from build123d import *

# Parameters (mm, degrees)
CROQUIS1_W              = 48
CROQUIS1_H              = 46
SALIENTE_EXTRUIR1_DEPTH = 26
CROQUIS2_W              = 44
CROQUIS2_H              = 22
CORTAR_EXTRUIR1_DEPTH   = 46
CROQUIS3_W              = 12.57
CROQUIS3_H              = 22
CORTAR_EXTRUIR3_DEPTH   = 60.236812878
REDONDEO3_R             = 10
REDONDEO4_R             = 10
CROQUIS16_W             = 12.57
CROQUIS16_H             = 4
CORTAR_EXTRUIR19_DEPTH  = 10.25
CROQUIS21_W             = 12.57
CROQUIS21_H             = 4
CORTAR_EXTRUIR20_DEPTH  = 10.25
CORTAR_EXTRUIR21_DEPTH  = 10.25
CROQUIS23_R             = 2.5
CORTAR_EXTRUIR22_DEPTH  = 53


with BuildPart() as part:
    # Croquis1 → Saliente-Extruir1 (new body)
    with BuildSketch(Plane(origin=(0, 0, 0), x_dir=(1, 0, 0), z_dir=(0, 1, 0))):
        Rectangle(CROQUIS1_W, CROQUIS1_H)
    extrude(amount=-SALIENTE_EXTRUIR1_DEPTH)

    # Croquis2 → Cortar-Extruir1 (cut)
    with BuildSketch(Plane.XY.offset(23)):
        with Locations((0, -15)):
            Rectangle(CROQUIS2_W, CROQUIS2_H)
    extrude(amount=-CORTAR_EXTRUIR1_DEPTH, mode=Mode.SUBTRACT)

    # Croquis3 → Cortar-Extruir3 (cut, through all)
    with BuildSketch(Plane(origin=(24, 0, 0), x_dir=(0, 0, -1), z_dir=(1, 0, 0))):
        with Locations((-16.715, -15)):
            Rectangle(CROQUIS3_W, CROQUIS3_H)
        with Locations((16.715, -15)):
            Rectangle(CROQUIS3_W, CROQUIS3_H)
    extrude(amount=-CORTAR_EXTRUIR3_DEPTH, mode=Mode.SUBTRACT)

    # Redondeo3
    redondeo3_edges = [part.edges().sort_by_distance(p)[0] for p in [
        (23, -26, 10.43),
        (23, -26, -10.43),
    ]]
    fillet(redondeo3_edges, radius=REDONDEO3_R)

    # Redondeo4
    redondeo4_edges = [part.edges().sort_by_distance(p)[0] for p in [
        (-23, -26, 10.43),
        (-23, -26, -10.43),
    ]]
    fillet(redondeo4_edges, radius=REDONDEO4_R)

    # Croquis16 → Cortar-Extruir19 (cut)
    with BuildSketch(Plane.ZY.offset(24)):
        with Locations((-16.715, -2)):
            Rectangle(CROQUIS16_W, CROQUIS16_H)
        with Locations((16.715, -2)):
            Rectangle(CROQUIS16_W, CROQUIS16_H)
    extrude(amount=-CORTAR_EXTRUIR19_DEPTH, mode=Mode.SUBTRACT)

    # Croquis21 → Cortar-Extruir20 (cut)
    with BuildSketch(Plane(origin=(24, 0, 0), x_dir=(0, 0, -1), z_dir=(1, 0, 0))):
        with Locations((-16.715, -2)):
            Rectangle(CROQUIS21_W, CROQUIS21_H)
        with Locations((16.715, -2)):
            Rectangle(CROQUIS21_W, CROQUIS21_H)
    extrude(amount=-CORTAR_EXTRUIR20_DEPTH, mode=Mode.SUBTRACT)

    # Croquis22 → Cortar-Extruir21 (cut)
    with BuildSketch(Plane(origin=(0, 0, 0), x_dir=(1, 0, 0), z_dir=(0, 1, 0))):
        with BuildLine():
            Line((13.75, -10.43), (13.75, -23))
            Line((13.75, -23), (-13.75, -23))
            Line((-13.75, -23), (-13.75, -10.43))
            ThreePointArc((-13.75, -10.43), (0, -17.258255995), (13.75, -10.43))
        make_face()
        with BuildLine():
            Line((13.75, 10.43), (13.75, 23))
            Line((13.75, 23), (-13.75, 23))
            Line((-13.75, 23), (-13.75, 10.43))
            ThreePointArc((-13.75, 10.43), (0, 17.258255995), (13.75, 10.43))
        make_face()
    extrude(amount=-CORTAR_EXTRUIR21_DEPTH, mode=Mode.SUBTRACT)

    # Croquis23 → Cortar-Extruir22 (cut)
    with BuildSketch(Plane.ZY.offset(24)):
        with Locations(Location((0, -21, 0), (0, 0, 180))):
            Circle(CROQUIS23_R)
    extrude(amount=-CORTAR_EXTRUIR22_DEPTH, mode=Mode.SUBTRACT)


solid = part.part
Part model, mm, in its own coordinate system. A direction names the side the tool comes from. Round coordinates to 2 decimals unless told otherwise and drop trailing zeros. Write each loop counter-clockwise with the first axis right and the second up, starting at its lowest first coordinate (ties: lowest second). Pieces come first, ordered by that corner, then holes. Notation, with made-up numbers: M 38,-31 L 59,-31 A13 ccw 59,-7 Z; hole C 43,59.25 d7. An arc over 180 degrees is marked long. Return JSON: item names as keys, results as strings. Group by question number.
(1) Pin check, flat tips, straight feed: pin 1 Ø8 at (x, y) = (-19.5, -4.5) entering from -Z; pin 2 Ø17.5 at (x, z) = (1.5, 2.5) entering from -Y; pin 3 Ø12 at (x, y) = (-11, -5.5) entering from +Z. Stop position of each tip, or through.
(2) Two-plate mould, pull along X, no slides. Class faces 1 (the face through (-22, -15, 0)), 2 (the face through (-0.223, -1.972, -17.257)), 3 (the face through (22.99, -22.99, 7.58)): +X half, -X half, draft (parallel to the pull), parting line (faces both ways), or undercut.
(3) Saw through at D-D on x = -18. Write the cut outline in (y, z), then the cut area to 3 significant figures.
(4) Which spindle directions (+Z, -Z, +X, -X, +Y, -Y) get a long thin tool onto all of the face, cutting with end or side? Do faces 4 (the face through (0, -4, 0)), 5 (the face through (-22.4, -4.6, -10.43)), 6 (the face through (-22.2, -4.6, 10.43)). Say none if no direction does.
(5) Drill centre lines: probe 1 along X at (y, z) = (-18.5, 5); probe 2 along Y at (x, z) = (22.45, 0); probe 3 along Y at (x, z) = (8.5, -11). Where is each one in solid material? Low to high.
(6) Saw through at A-A on y = -9.25. Write the cut outline in (x, z).
(7) Saw through at C-C on y = -21. Write the cut outline in (x, z).
(8) Saw through at B-B on z = 1.5. Write the cut outline in (x, y), then the cut area to 3 significant figures.
Returned:
{
 "1": {"pin 1": "z = -10.43", "pin 2": "y = -4", "pin 3": "z = 16.46"},
 "2": {"face 1": "undercut", "face 2": "parting line", "face 3": "draft"},
 "3": {"outline": "M -4,-10.43 L 0,-10.43 L 0,10.43 L -4,10.43 Z", "area": "83.4 mm²"},
 "4": {"face 4": "+Z, -Z, -Y", "face 5": "-Z, -X, +Y, -Y", "face 6": "+Z, -X, +Y, -Y"},
 "5": {"probe 1": "-24 to -22, 22 to 24", "probe 2": "-26 to -23.5, -18.5 to 0", "probe 3": "-4 to 0"},
 "6": {"outline": "M -24,-10.43 L -22,-10.43 L -22,10.43 L -24,10.43 Z; M 22,-10.43 L 24,-10.43 L 24,10.43 L 22,10.43 Z"},
 "7": {"outline": "M -24,-9.09 L -22,-9.09 L -22,-2.5 L -24,-2.5 Z; M -24,2.5 L -22,2.5 L -22,9.09 L -24,9.09 Z; M 22,-9.09 L 24,-9.09 L 24,-2.5 L 22,-2.5 Z; M 22,2.5 L 24,2.5 L 24,9.09 L 22,9.09 Z"},
 "8": {"outline": "M -24,-25.94 L -22,-25.94 L -22,-23 L -24,-23 Z; M -24,-19 L -22,-19 L -22,-4 L 22,-4 L 22,-19 L 24,-19 L 24,0 L -24,0 Z; M 22,-25.94 L 24,-25.94 L 24,-23 L 22,-23 Z", "area": "264 mm²"}
}
